Autodesk Inventor part; units mm, degrees
ref_plane "YZ Plane" through (0, 0, 0) normal (1, 0, 0) x (0, 1, 0)
ref_plane "XZ Plane" through (0, 0, 0) normal (0, 1, 0) x (-1, 0, 0)
ref_plane "XY Plane" through (0, 0, 0) normal (0, 0, 1) x (1, 0, 0)
sketch "草圖2" plane through (0, 0, 0) normal (0, 1, 0) x (-1, 0, 0)
  line L0 (0, 0) -> (19.2, 0)
  line L1 (19.2, 0) -> (19.2, -26.2)
  line L2 (19.2, -26.2) -> (0, -26.2)
  line L3 (0, -26.2) -> (0, 0)
  dimension "d4" = 26.2
  dimension "d5" = 19.2
extrude "擠出2" add sketch "草圖2" along normal blind 1.5
sketch "草圖3" plane through (0, 1.5, 0) normal (0, 1, 0) x (1, 0, 0)
  line L0 (-19.2, 0) -> (0, 0)
  line L1 (-19.2, 26.2) -> (-19.2, 0)
  line L2 (-17.2, 4.5) -> (-5.2, 4.5)
  line L3 (-5.2, 4.5) -> (-5.2, 16.5)
  line L4 (-5.2, 16.5) -> (-17.2, 16.5)
  line L5 (-17.2, 16.5) -> (-17.2, 4.5)
  dimension "d8" = 4.5
  dimension "d9" = 2
  dimension "d10" = 12
  dimension "d11" = 12
extrude "擠出3" add sketch "草圖3" along normal blind 6.6
sketch "草圖4" plane through (0, 8.1, 0) normal (0, 1, 0) x (1, 0, 0)
  line L0 (-5.2, 4.5) -> (-5.2, 16.5)
  line L1 (-5.2, 16.5) -> (-17.2, 16.5)
  line L2 (-17.2, 16.5) -> (-17.2, 4.5)
  line L3 (-17.2, 4.5) -> (-5.2, 4.5)
  circle A0 centre (-11.2, 10.5) radius 3.4
  point P0 (0, 0)
  dimension "d14" = 6
  dimension "d15" = 6
  dimension "d16" = 6.8
extrude "擠出4" add sketch "草圖4" along normal blind 7.46 contours A0
sketch "草圖5" plane through (-11.2, 15.56, -10.5) normal (0, 1, 0) x (1, 0, 0)
  circle A0 centre (0, 0) radius 3.4
  circle A1 centre (0, 0) radius 3
  point P0 (11.2, -10.5)
  dimension "d19" = 6
extrude "擠出5" add sketch "草圖5" along normal blind 12.54 contours A1
thread "螺紋1"
sketch "草圖6" plane through (-11.2, 28.1, -10.5) normal (0, 1, 0) x (1, 0, 0)
  line L0 (-3, 1.4) -> (3, 1.4)
  line L1 (3, 1.4) -> (3, 3)
  line L2 (3, 3) -> (-3, 3)
  line L3 (-3, 3) -> (-3, 1.4)
  circle A0 centre (0, 0) radius 3
  point P0 (11.2, -10.5)
  point P1 (0, 3)
  point P2 (0, 3)
  point P3 (-3, 0)
  dimension "d24" = 1.6
  dimension "d25" = 6
extrude "擠出6" cut sketch "草圖6" against normal blind 10 contours L3 L2 A0 L0 | A0 L0 | A0 L2 L1 L0 picked at (0.7632, 1.5795)
sketch "草圖7" plane through (0, 0, 0) normal (0, -1, 0) x (1, 0, 0)
  circle A0 centre (-2.4, -4.7) radius 1.4
  circle A1 centre (-2.4, -21.5) radius 1.4
  line L0 (0, 0) -> (0, -26.2)
  line L1 (-19.2, 0) -> (0, 0)
  dimension "d29" = 16.8
  dimension "d30" = 2.8
  dimension "d31" = 2.4
  dimension "d33" = 4.7
extrude "擠出7" cut sketch "草圖7" against normal up to surface (1.5 mm away)
properties part number "編碼器"
Geometry check sheet. Reference: the model listing, model coordinates, mm. A direction names the side the tool comes from. Coordinates: 2 decimals unless noted, no trailing zeros. Order: outer loops, then holes, each group sorted by start corner. A loop starts at its lowest first (then second) coordinate and runs counter-clockwise, first axis right, second up. Notation, with made-up numbers: M -39,13 L -28,13 A16 cw -28,17 Z; hole C -22.75,84 d2. An arc over 180 degrees is marked long. Answer as a JSON object with one key per item and string values.
Q1. Scan lines: line 1 (Z direction, x = -2.4, y = 0.6); line 2 (Z direction, x = -6, y = 6); line 3 (Y direction, x = -2.75, z = -20). Record each from-to range of solid material in increasing order.
Results are:
{"line 1": "z = -26.2 to -22.9, -20.1 to -6.1, -3.3 to 0", "line 2": "z = -16.5 to -4.5", "line 3": "y = 0 to 1.5"}
Q2. Release check for a two-part mould opening along X. For faces 5 (the flat face through (-11, 18.1, -13)), 6 (the cylindrical face through (-3.43, 0.74, -3.75)), 7 (the flat face through (-5.2, 5, -10)), 8 (the cylindrical face through (-2.703, 0.74, -22.867)) record: released by +X, released by -X, zero draft, split by the parting line, or undercut.
Results are:
{"face 5": "zero draft", "face 6": "undercut", "face 7": "released by +X", "face 8": "undercut"}
Q3. Cross-section at D-D on x = -2.25. Record the cut outline in (y, z).
Results are:
{"outline": "M 0,-26.2 L 1.5,-26.2 L 1.5,-22.89 L 0,-22.89 Z; M 0,-20.11 L 1.5,-20.11 L 1.5,-6.09 L 0,-6.09 Z; M 0,-3.31 L 1.5,-3.31 L 1.5,0 L 0,0 Z"}
Q4. Cross-section at B-B on x = -11.2. Record the cut outline in (y, z).
Results are:
{"outline": "M 0,-26.2 L 1.5,-26.2 L 1.5,-16.5 L 8.1,-16.5 L 8.1,-13.9 L 15.56,-13.9 L 15.56,-13.5 L 18.1,-13.5 L 18.1,-11.9 L 28.1,-11.9 L 28.1,-7.5 L 15.56,-7.5 L 15.56,-7.1 L 8.1,-7.1 L 8.1,-4.5 L 1.5,-4.5 L 1.5,0 L 0,0 Z"}
Q5. Cross-section at A-A on z = -21.5. Record the cut outline in (x, y).
Results are:
{"outline": "M -19.2,0 L -3.8,0 L -3.8,1.5 L -19.2,1.5 Z; M -1,0 L 0,0 L 0,1.5 L -1,1.5 Z"}
Q6. Depth check by flat-ended pin: pin 1 Ø3.5 at (x, y) = (-10.5, 5) entering from -Z; pin 2 Ø2 at (y, z) = (6, -11) entering from -X; pin 3 Ø1 at (x, y) = (-10.5, 25) entering from -Z. Enter the tip coordinate at first touch or a pass-through.
Results are:
{"pin 1": "stops at z = -16.5", "pin 2": "stops at x = -17.2", "pin 3": "stops at z = -11.9"}
Q7. Tool access check on faces 1 (the flat face through (-11, 5, -4.5)), 2 (the flat face through (-11, 28.1, -10)), 3 (the cylindrical face through (-11.591, 21.742, -7.526)), 4 (the flat face through (-11, 5, -16.5)). Record the directions out of +Z, -Z, +X, -X, +Y, -Y that give a thin tool (end or side, any length) a straight path to the whole face; none if there is none.
Results are:
{"face 1": "+Z, +X, -X, +Y", "face 2": "+Z, -Z, +X, -X, +Y", "face 3": "+Y", "face 4": "-Z, +X, -X, +Y"}
Q8. Cross-section at C-C on z = -15. Record the cut outline in (x, y), and give its area (3 significant figures).
Results are:
{"outline": "M -19.2,0 L 0,0 L 0,1.5 L -5.2,1.5 L -5.2,8.1 L -17.2,8.1 L -17.2,1.5 L -19.2,1.5 Z", "area": "108 mm²"}
